```python
from build123d import *

# Parameters (mm, degrees)
F0_R     = 15
F1_DEPTH = 90
F2_R     = 1.5
F3_DEPTH = 25
F4_R     = 5


with BuildPart() as f1:
    # F0 (on Top) → F1 (new body)
    with BuildSketch(Plane.XY):
        Circle(F0_R)
    extrude(amount=F1_DEPTH)

    # F2 (on face) → F3 (cut)
    with BuildSketch(Plane.XY.offset(90)):
        Circle(F2_R)
    extrude(amount=-F3_DEPTH, mode=Mode.SUBTRACT)

    # F4
    f4_edges = [f1.edges().sort_by_distance(p)[0] for p in [
        (-15, 0, 0),
    ]]
    fillet(f4_edges, radius=F4_R)


solid = f1.part
```
Model file for the job. Use its own axes, mm. A direction names the side the tool comes from. Coordinates: 2 decimals unless noted, no trailing zeros. Order: outer loops, then holes, each group sorted by start corner. A loop starts at its lowest first (then second) coordinate and runs counter-clockwise, first axis right, second up. Notation, with made-up numbers: (60, 38.25) -> (87, 38.25) arc R23 ccw to (87, 65.25) -> close; hole circle Ø8 at (69.5, 33). An arc over 180 degrees is marked (long way). Return JSON: item names as keys, results as strings.
Item 1: Mould opens along X. For faces 1 (the face through (0, 0, 65)), 2 (the face through (0, 0, 0)), 3 (the face through (-14.985, 0.66, 46.905)) say: pulls with the +X half, pulls with the -X half, needs draft (parallel to the pull), parting line crosses it, or undercut.
Model answer:
{"face 1": "undercut", "face 2": "needs draft", "face 3": "parting line crosses it"}
Item 2: Slice it at C-C (z = 48). Write the cut outline in (x, y), then the cut area to 3 significant figures.
Model answer:
{"outline": "circle Ø30 at (0, 0)", "area": "707 mm²"}
Item 3: 3-axis set-ups, long thin cutter, end or side, ignore diameter. For faces 4 (the face through (-1.5, 0.07, 77.68)), 5 (the face through (3, 0, 90)): which of +Z, -Z, +X, -X, +Y, -Y reach the whole face in a straight line?
Model answer:
{"face 4": "+Z", "face 5": "+Z, +X, -X, +Y, -Y"}
Item 4: Slice it at D-D (z = 80). Write the cut outline in (x, y), then the cut area to 3 significant figures.
Model answer:
{"outline": "circle Ø30 at (0, 0); hole circle Ø3 at (0, 0)", "area": "700 mm²"}
Item 5: Wall check: line 1 along Y through (x, z) = (0, 70); line 2 along Z through (x, y) = (5.5, 8.75); line 3 along Z through (x, y) = (13.5, 0.5). Give the ranges that are in metal, low to high. Write a range as from..to.
Model answer:
{"line 1": "y = -15..-1.5, 1.5..15", "line 2": "z = 0.01..90", "line 3": "z = 1.44..90"}
Item 6: Slice it at A-A (y = 0). Write the cut outline in (x, z), then the cut area to 3 significant figures.
Model answer:
{"outline": "(-15, 5) arc R5 ccw to (-10, 0) -> (10, 0) arc R5 ccw to (15, 5) -> (15, 90) -> (1.5, 90) -> (1.5, 65) -> (-1.5, 65) -> (-1.5, 90) -> (-15, 90) -> close", "area": "2,610 mm²"}
Item 7: Pin check, flat tips, straight feed: P1, Ø2.5, axis at x = 0, y = 0, coming from the +Z side; P2, Ø1, axis at x = -8.5, z = 38, coming from the -Y side; P3, Ø12, axis at x = -10, z = 76, coming from the +Y side; P4, Ø6, axis at x = 4, y = 12, coming from the -Z side. Stop position of each tip, or through.
Model answer:
{"P1": "stops at z = 65", "P2": "stops at y = -12.69", "P3": "stops at y = 14.46", "P4": "stops at z = 0"}
